Read the model definition and answer for the solid it produces. Units are mm, in the model's axes. Face numbers are marked on the shaded views. Give positions to 0.01 mm unless a question says otherwise; leave off trailing zeros. Write each loop counter-clockwise with the first axis right and the second up, starting at its lowest first coordinate (ties: lowest second). Pieces come first, ordered by that corner, then holes. Notation, with made-up numbers: (31, 34.25) -> (76, 34.25) arc R9 cw to (76, 51.25) -> close; hole circle Ø4 at (57.5, -10.5). An arc over 180 degrees is marked (long way). Write item = value, one per line.
from build123d import *

# Parameters (mm, degrees)
SKETCH070_R  = 6.5
PAD_DEPTH    = 1.2
SKETCH069_R  = 5.8
PAD001_DEPTH = 5.6
SKETCH071_R  = 5
POCKET_DEPTH = 3.5
FILLET_R     = 1


with BuildPart() as part:
    # Sketch070 → Pad (new body)
    with BuildSketch(Plane.XZ):
        Circle(SKETCH070_R)
    extrude(amount=PAD_DEPTH)

    # Sketch069 → Pad001 (join)
    with BuildSketch(Plane.XZ):
        Circle(SKETCH069_R)
    extrude(amount=PAD001_DEPTH)

    # Sketch071 → Pocket (cut, symmetric)
    with BuildSketch(Plane.XZ):
        Circle(SKETCH071_R)
    extrude(amount=POCKET_DEPTH, both=True, mode=Mode.SUBTRACT)

    # Fillet
    fillet_edges = [part.edges().sort_by_distance(p)[0] for p in [
        (-5.8, -5.6, 0),
    ]]
    fillet(fillet_edges, radius=FILLET_R)


solid = part.part
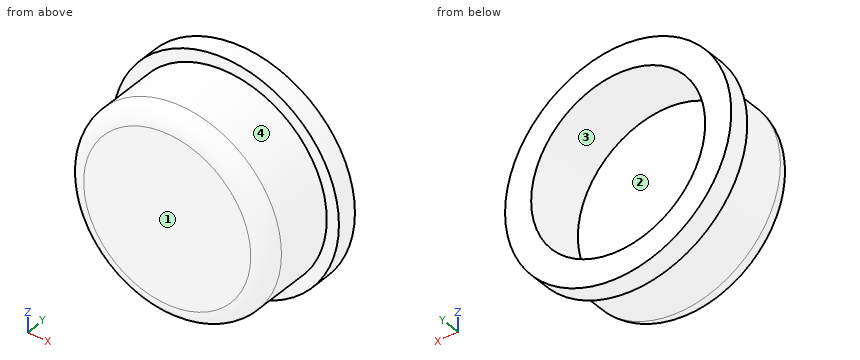
(1) For a pull along Z with two mould halves and no side action, classify the marked faces 1, 2, 3 and 4 as released by +Z, released by -Z, zero draft, split by the parting line, or undercut.
Checks:
face_1 = zero draft
face_2 = undercut
face_3 = undercut
face_4 = split by the parting line
(2) The part is cut by section A-A on z = 0. Determine the outline of the cut face in (x, y), plus the area to 3 significant figures.
Checks:
outline = (-6.5, -1.2) -> (-5.8, -1.2) -> (-5.8, -4.6) arc R1 ccw to (-4.8, -5.6) -> (4.8, -5.6) arc R1 ccw to (5.8, -4.6) -> (5.8, -1.2) -> (6.5, -1.2) -> (6.5, 0) -> (5, 0) -> (5, -3.5) -> (-5, -3.5) -> (-5, 0) -> (-6.5, 0) -> close
area = 31.2 mm²
(3) The part is cut by section C-C on y = -0.35. Determine the outline of the cut face in (x, z).
Checks:
outline = circle Ø13 at (0, 0); hole circle Ø10 at (0, 0)
(4) The part is cut by section D-D on y = -1.45. Determine the outline of the cut face in (x, z), plus the area to 3 significant figures.
Checks:
outline = circle Ø11.6 at (0, 0); hole circle Ø10 at (0, 0)
area = 27.1 mm²
(5) The part is cut by section B-B on x = 0. Determine the outline of the cut face in (y, z), plus the area to 3 significant figures.
Checks:
outline = (-5.6, -4.8) arc R1 ccw to (-4.6, -5.8) -> (-1.2, -5.8) -> (-1.2, -6.5) -> (0, -6.5) -> (0, -5) -> (-3.5, -5) -> (-3.5, 5) -> (0, 5) -> (0, 6.5) -> (-1.2, 6.5) -> (-1.2, 5.8) -> (-4.6, 5.8) arc R1 ccw to (-5.6, 4.8) -> close
area = 31.2 mm²
(6) Consider L1, parallel to X at y = -3.3, z = 0.5; L2, parallel to Y at x = 3.25, z = 2.75; L3, parallel to Z at x = 0, y = -1.9. Determine where each line is inside the solid, lowest interval first.
Checks:
L1 = -5.78 to -4.97, 4.97 to 5.78
L2 = -5.6 to -3.5
L3 = -5.8 to -5, 5 to 5.8
(7) Given P1, Ø2, axis at y = -0.5, z = -3, coming from the +X side; P2, Ø1, axis at x = -0.5, y = -5, coming from the +Z side, each flat-ended and moving along its own axis, determine where each tip first touches the part or whether it passes through.
Checks:
P1 = 6.18
P2 = 5.8
